Geometry check sheet. Reference: the model listing, model coordinates, mm. Face numbers are marked on the shaded views. Round coordinates to 2 decimals unless told otherwise and drop trailing zeros. Order: outer loops, then holes, each group sorted by start corner. A loop starts at its lowest first (then second) coordinate and runs counter-clockwise, first axis right, second up.
```python
from build123d import *

# Parameters (mm, degrees)
F3_DEPTH = 943


with BuildPart() as f3:
    # F2 (on face) → F3 (new body, through all)
    with BuildSketch(Plane.XZ.offset(471.5)):
        with BuildLine():
            ThreePointArc((-2.5, -92), (-0.732233, -91.267767), (0, -89.5))
            Line((0, -89.5), (0, 89.5))
            ThreePointArc((0, 89.5), (-0.732233, 91.267767), (-2.5, 92))
            Line((-2.5, 92), (-51, 92))
            Line((-51, 92), (-51, 87.5))
            Line((-51, 87.5), (-7, 87.5))
            ThreePointArc((-7, 87.5), (-5.232233, 86.767767), (-4.5, 85))
            Line((-4.5, 85), (-4.5, -85))
            ThreePointArc((-4.5, -85), (-5.232233, -86.767767), (-7, -87.5))
            Line((-7, -87.5), (-51, -87.5))
            Line((-51, -87.5), (-51, -92))
            Line((-51, -92), (-2.5, -92))
        make_face()
    extrude(amount=-F3_DEPTH)


solid = f3.part
```
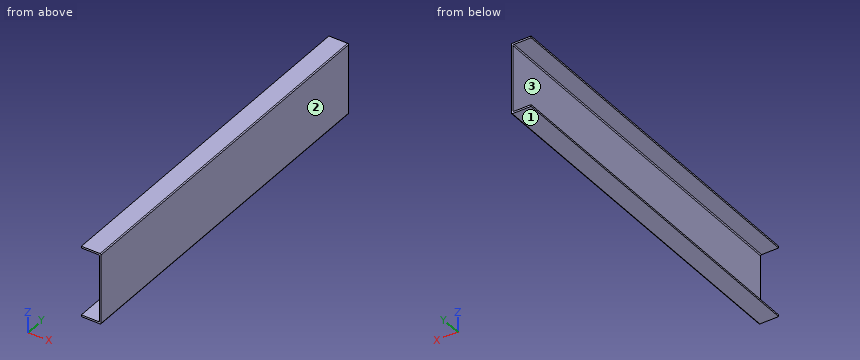
(1) Depth check by flat-ended pin: P1, Ø10, axis at y = 342, z = 5.5, coming from the -X side. Enter the tip coordinate at first touch or a pass-through.
Returned:
P1: stops at x = -4.5
(2) Material ranges on line 1 (Z direction, x = -45, y = -1.5); line 2 (X direction, y = -107, z = 28), recorded low to high.
Returned:
line 1: z = -92 to -87.5, 87.5 to 92
line 2: x = -4.5 to 0
(3) Draft check along Z on the marked faces 1, 2 and 3. Enter one of: released by +Z, released by -Z, zero draft, split by the parting line, or undercut.
Returned:
face 1: released by -Z
face 2: zero draft
face 3: undercut
(4) Sectioned sample at C-C, the plane z = -33. Record the cut outline in (x, y), and give its area (3 significant figures).
Returned:
outline: (-4.5, -471.5) - (0, -471.5) - (0, 471.5) - (-4.5, 471.5) - close
area: 4,240 mm2
(5) Sectioned sample at A-A, the plane x = -40. Record the cut outline in (y, z), and give its area (3 significant figures).
Returned:
outline: (-471.5, -92) - (471.5, -92) - (471.5, -87.5) - (-471.5, -87.5) - close; (-471.5, 87.5) - (471.5, 87.5) - (471.5, 92) - (-471.5, 92) - close
area: 8,490 mm2
(6) Sectioned sample at B-B, the plane y = 130.5. Record the cut outline in (x, z).
Returned:
outline: (-51, -92) - (-2.5, -92) arc R2.5 ccw to (0, -89.5) - (0, 89.5) arc R2.5 ccw to (-2.5, 92) - (-51, 92) - (-51, 87.5) - (-7, 87.5) arc R2.5 cw to (-4.5, 85) - (-4.5, -85) arc R2.5 cw to (-7, -87.5) - (-51, -87.5) - close
